from build123d import *

# Parameters (mm, degrees)
SKETCH1_R                 = 12.7
BOSS_EXTRUDE1_DEPTH       = 3.175
SKETCH2_R                 = 6.35
BOSS_EXTRUDE2_DEPTH       = 22.225
SKETCH3_R                 = 3
CUT_EXTRUDE1_DEPTH        = 3.175
SKETCH4_R                 = 3.96875
CUT_EXTRUDE2_DEPTH        = 19.05
CUT_EXTRUDE3_REACH        = 8.35
SKETCH5_R                 = 1.6
F_6_32_TAPPED_HOLE1_D     = 2.7051
F_6_32_TAPPED_HOLE1_DEPTH = 3.175


with BuildPart() as part:
    # Sketch1 → Boss-Extrude1 (new body)
    with BuildSketch(Plane(origin=(0, 0, 0), x_dir=(1, 0, 0), z_dir=(0, 1, 0))):
        Circle(SKETCH1_R)
    extrude(amount=BOSS_EXTRUDE1_DEPTH)

    # Sketch2 → Boss-Extrude2 (add)
    with BuildSketch(Plane(origin=(0, 0, 0), x_dir=(1, 0, 0), z_dir=(0, 1, 0))):
        Circle(SKETCH2_R)
    extrude(amount=-BOSS_EXTRUDE2_DEPTH)

    # Sketch3 → Cut-Extrude1 (cut)
    with BuildSketch(Plane.XZ.offset(22.225)):
        Circle(SKETCH3_R)
    extrude(amount=-CUT_EXTRUDE1_DEPTH, mode=Mode.SUBTRACT)

    # Sketch4 → Cut-Extrude2 (cut)
    with BuildSketch(Plane(origin=(0, 3.175, 0), x_dir=(1, 0, 0), z_dir=(0, 1, 0))):
        Circle(SKETCH4_R)
    extrude(amount=-CUT_EXTRUDE2_DEPTH, mode=Mode.SUBTRACT)

    # Sketch5 → Cut-Extrude3 (cut, up to next)
    with BuildSketch(Plane(origin=(0, -15.875, 0), x_dir=(1, 0, 0), z_dir=(0, 1, 0)), mode=Mode.PRIVATE) as cut_extrude3_sk1:
        Circle(SKETCH5_R)
    cut_extrude3_tool1 = extrude(cut_extrude3_sk1.sketch, amount=-CUT_EXTRUDE3_REACH, mode=Mode.PRIVATE) & part.part
    add(cut_extrude3_tool1.solids().sort_by_distance((0, -15.875, 0))[0], mode=Mode.SUBTRACT)

    # #6-32 Tapped Hole1
    with Locations(Plane(origin=(0, 3.175, 0), x_dir=(-1, 0, 0), z_dir=(0, 1, 0))):
        with Locations((0, -9.779), (-6.914797213, -6.914797213), (-9.779, 0), (-6.914797213, 6.914797213), (0, 9.779), (6.914797213, 6.914797213), (9.779, 0), (6.914797213, -6.914797213)):
            Hole(F_6_32_TAPPED_HOLE1_D / 2, depth=F_6_32_TAPPED_HOLE1_DEPTH)


solid = part.part
CAD build for the part. Positions are in the model's coordinates, mm. A direction names the side the tool comes from. Give positions to 0.01 mm unless a question says otherwise; leave off trailing zeros. Write each loop counter-clockwise with the first axis right and the second up, starting at its lowest first coordinate (ties: lowest second). Pieces come first, ordered by that corner, then holes. Notation, with made-up numbers: M 79,36 L 97,36 A31 ccw 97,60 Z; hole C -38.5,58.25 d7. An arc over 180 degrees is marked long. Put each result on its own line as item: value. Start each with the question number.
(1) Mould opens along Z. For faces 4 (the face through (3, 0, -6)), 5 (the face through (-2.75, 1.57, 12.4)), 6 (the face through (-11.13, 1.57, 0.06)) say: +Z half, -Z half, draft (parallel to the pull), parting line (faces both ways), or undercut.
(2) Probe L1, parallel to Z at x = 0, y = 1.3; L2, parallel to X at y = -7.5, z = 0; L3, parallel to Z at x = 0, y = -21. List the from-to ranges inside material, lowest first.
(3) Band-saw the part on C-C, the plane x = -7.5. Write the cut outline in (y, z) (3 decimals), and give its area (3 significant figures).
(4) Flat gauge pins, fed straight in: pin 1 Ø2 at (x, z) = (0, 9.779) entering from -Y; pin 2 Ø3 at (y, z) = (-7.5, -5.5) entering from +X; pin 3 Ø5.5 at (x, z) = (0, 0) entering from +Y (3 decimals); pin 4 Ø12 at (y, z) = (-14, 0.5) entering from -X. Where does each tip first touch, or does it go through?
(5) Band-saw the part on D-D, the plane y = -11.75. Write the cut outline in (x, z), and give its area (3 significant figures).
(6) Band-saw the part on B-B, the plane z = 0. Write the cut outline in (x, y) (3 decimals).
(7) Band-saw the part on A-A, the plane x = 0. Write the cut outline in (y, z) (3 decimals).
(8) Which spindle directions (+Z, -Z, +X, -X, +Y, -Y) get a long thin tool onto all of the face, cutting with end or side? Do faces 1 (the face through (-0.29, 1.57, -11.1)), 2 (the face through (2, -15.875, 0)), 3 (the face through (1.3, -19.05, -1.3)). Say none if no direction does.
Response values:
1. face 4: draft
1. face 5: parting line
1. face 6: undercut
2. L1: z = -12.7 to -11.13, -8.43 to -3.97, 3.97 to 8.43, 11.13 to 12.7
2. L2: x = -6.35 to -3.97, 3.97 to 6.35
2. L3: z = -6.35 to -3, 3 to 6.35
3. outline: M 0,-10.249 L 3.175,-10.249 L 3.175,-8.134 L 0,-8.134 Z; M 0,-5.695 L 3.175,-5.695 L 3.175,5.695 L 0,5.695 Z; M 0,8.134 L 3.175,8.134 L 3.175,10.249 L 0,10.249 Z
3. area: 49.6 mm2
4. pin 1: passes through
4. pin 2: stops at x = 4.93
4. pin 3: stops at y = -15.875
4. pin 4: stops at x = -6.35
5. outline: C 0,0 d12.7; hole C 0,0 d7.94
5. area: 77.2 mm2
6. outline: M -12.7,0 L -11.132,0 L -11.132,3.175 L -12.7,3.175 Z; M -8.426,0 L -6.35,0 L -6.35,-22.225 L -3,-22.225 L -3,-19.05 L -1.6,-19.05 L -1.6,-15.875 L -3.969,-15.875 L -3.969,3.175 L -8.426,3.175 Z; M 1.6,-19.05 L 3,-19.05 L 3,-22.225 L 6.35,-22.225 L 6.35,0 L 8.426,0 L 8.426,3.175 L 3.969,3.175 L 3.969,-15.875 L 1.6,-15.875 Z; M 11.132,0 L 12.7,0 L 12.7,3.175 L 11.132,3.175 Z
7. outline: M -22.225,-6.35 L 0,-6.35 L 0,-8.426 L 3.175,-8.426 L 3.175,-3.969 L -15.875,-3.969 L -15.875,-1.6 L -19.05,-1.6 L -19.05,-3 L -22.225,-3 Z; M -22.225,3 L -19.05,3 L -19.05,1.6 L -15.875,1.6 L -15.875,3.969 L 3.175,3.969 L 3.175,8.426 L 0,8.426 L 0,6.35 L -22.225,6.35 Z; M 0,-12.7 L 3.175,-12.7 L 3.175,-11.132 L 0,-11.132 Z; M 0,11.132 L 3.175,11.132 L 3.175,12.7 L 0,12.7 Z
8. face 1: +Y, -Y
8. face 2: +Y
8. face 3: -Y
